Geometry: see drawing. Coordinates: mm, zero at the bounding-box minimum. A direction names the side the tool comes from. Coordinates: 2 decimals unless noted, no trailing zeros. Order: outer loops, then holes, each group sorted by start corner. A loop starts at its lowest first (then second) coordinate and runs counter-clockwise, first axis right, second up.
Item 1: Ray query, line 1 (X direction, y = 1.1, z = 1.5); line 2 (Z direction, x = 21.5, y = 1.05); line 3 (Y direction, x = 13.5, z = 13.75). Return the intervals inside material, ascending.
Item 2: Section D-D on z = 1.5. Return the cut outline in (x, y), then the cut area to 3 significant figures.
Item 3: Section B-B on x = 21.5. State how many separate pieces and enclosed holes the cut face has, then the cut area to 3 significant figures.
Item 4: Mould query, pull axis Z, two halves, no side actions, for the marked faces 1, 2 and 3. Classes: released by +Z, released by -Z, zero draft, split by the parting line, or undercut.
Item 5: Section A-A on y = 1.5. Return the cut outline in (x, z).
Item 6: Section C-C on z = 7.25. Return the cut outline in (x, y), then the cut area to 3 significant figures.
Item 7: Contact query for flat-ended pins moving along their axis: P1, Ø7, axis at x = 15.5, z = 14, coming from the +Y side; P2, Ø0.9, axis at x = 15.5, y = 3.5, coming from the -Z side; P3, Ø10, axis at x = 12, z = 7.5, coming from the +Y side. Output: stop coordinate, or through.
Item 8: Reachability of the marked faces 4 and 5 from +Z, -Z, +X, -X, +Y, -Y: full face, straight path, thin tool, end or side. Return the list, or none.
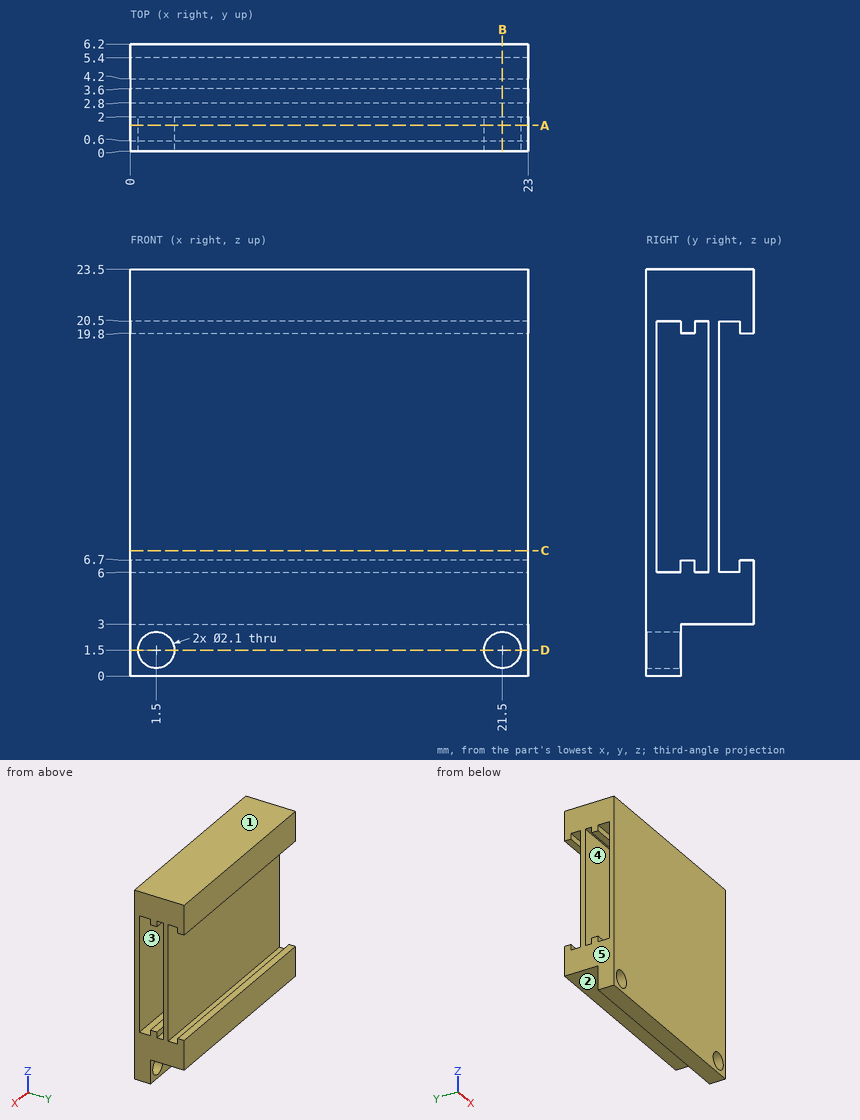
Answer list:
1. line 1: x = 0 to 0.45, 2.55 to 20.45, 22.55 to 23
1. line 2: z = 0 to 0.45, 2.55 to 6, 20.5 to 23.5
1. line 3: y = 0 to 0.6, 3.6 to 4.2
2. outline: (0, 0) - (0.45, 0) - (0.45, 2) - (0, 2) - close; (2.55, 0) - (20.45, 0) - (20.45, 2) - (2.55, 2) - close; (22.55, 0) - (23, 0) - (23, 2) - (22.55, 2) - close
2. area: 37.6 mm2
3. separate pieces: 2
3. enclosed holes: 1
3. area: 58.6 mm2
4. face 1: released by +Z
4. face 2: released by -Z
4. face 3: undercut
5. outline: (0, 0) - (23, 0) - (23, 6) - (0, 6) - close; (0, 20.5) - (23, 20.5) - (23, 23.5) - (0, 23.5) - close; hole circle Ø2.1 at (1.5, 1.5); hole circle Ø2.1 at (21.5, 1.5)
6. outline: (0, 0) - (23, 0) - (23, 0.6) - (0, 0.6) - close; (0, 3.6) - (23, 3.6) - (23, 4.2) - (0, 4.2) - close
6. area: 27.6 mm2
7. P1: stops at y = 4.2
7. P2: stops at z = 3
7. P3: stops at y = 6.2
8. face 4: +X, -X
8. face 5: +Z, -Z, -X, +Y, -Y
